For this review, take the finished solid that the model builds, in its own axes (mm). Face numbers are marked on the shaded views. A direction names the side the tool comes from. Give positions to 0.01 mm unless a question says otherwise; leave off trailing zeros. Write each loop counter-clockwise with the first axis right and the second up, starting at its lowest first coordinate (ties: lowest second). Pieces come first, ordered by that corner, then holes. Notation, with made-up numbers: (68.5, -27) -> (80.5, -27) arc R22 ccw to (80.5, -19) -> close; hole circle Ø4 at (21.25, -31.75). An arc over 180 degrees is marked (long way). Return JSON: item names as keys, results as strings.
from build123d import *

# Parameters (mm, degrees)
EKSTR_ZYON_NCE1_DEPTH = 50
IZIM2_R               = 3
KES_EKSTR_ZYON1_DEPTH = 78
IZIM3_R               = 0.5
KES_EKSTR_ZYON2_DEPTH = 22
IZIM4_R               = 6
KES_EKSTR_ZYON3_DEPTH = 22


with BuildPart() as part:
    # Çizim1 → Ekstrüzyon-İnce1 (new body)
    with BuildSketch(Plane.XY):
        with BuildLine():
            Line((0, 0), (0, 29))
            ThreePointArc((0, 29), (0.292893219, 29.707106781), (1, 30))
            Line((1, 30), (57, 30))
            ThreePointArc((57, 30), (57.707106781, 29.707106781), (58, 29))
            Line((58, 29), (58, 0))
            Line((58, 0), (57, 0))
            Line((57, 0), (57, 29))
            Line((57, 29), (1, 29))
            Line((1, 29), (1, 0))
            Line((1, 0), (0, 0))
        make_face()
    extrude(amount=EKSTR_ZYON_NCE1_DEPTH)

    # Çizim2 → Kes-Ekstrüzyon1 (cut)
    with BuildSketch(Plane(origin=(58, 0, 0), x_dir=(0, 0, -1), z_dir=(1, 0, 0))):
        with Locations((-36.75, 14.5)):
            Circle(IZIM2_R)
        with Locations((-13.25, 14.5)):
            Circle(IZIM2_R)
    extrude(amount=-KES_EKSTR_ZYON1_DEPTH, mode=Mode.SUBTRACT)

    # Çizim3 → Kes-Ekstrüzyon2 (cut)
    with BuildSketch(Plane.ZY):
        with Locations((46.926319902, 2.636193895)):
            Circle(IZIM3_R)
    extrude(amount=-KES_EKSTR_ZYON2_DEPTH, mode=Mode.SUBTRACT)

    # Çizim4 → Kes-Ekstrüzyon3 (cut)
    with BuildSketch(Plane.ZY):
        with Locations((36.75, 14.5)):
            Circle(IZIM4_R)
    extrude(amount=-KES_EKSTR_ZYON3_DEPTH, mode=Mode.SUBTRACT)


solid = part.part
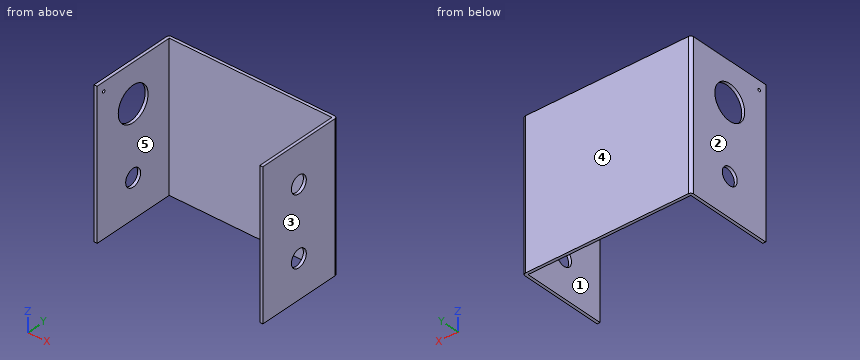
1. The part is to be moulded in two halves that separate along X. For the marked faces 1, 2 and 3, say which applies: +X half, -X half, draft (parallel to the pull), parting line (faces both ways), or undercut.
Results found:
{"face 1": "undercut", "face 2": "-X half", "face 3": "+X half"}
2. For pin 1 (1.5 mm diameter, centred on x = 22, z = 10.5, fed in from -Y), flat-tipped, find the tip position at first contact; note if it passes through.
Results found:
{"pin 1": "stops at y = 29"}
3. Add section C-C, the plane z = 13.25. State the section outline as (x, y) points, plus the area to 3 significant figures.
Results found:
{"outline": "(0, 0) -> (1, 0) -> (1, 11.5) -> (0, 11.5) -> close; (0, 17.5) -> (1, 17.5) -> (1, 29) -> (57, 29) -> (57, 17.5) -> (58, 17.5) -> (58, 29) arc R1 ccw to (57, 30) -> (1, 30) arc R1 ccw to (0, 29) -> close; (57, 0) -> (58, 0) -> (58, 11.5) -> (57, 11.5) -> close", "area": "104 mm²"}
4. For the marked faces 4 and 5, list the 3-axis set-ups (+Z, -Z, +X, -X, +Y, -Y) from which the entire face can be reached by the end or side of a thin tool; tool diameter is ignored.
Results found:
{"face 4": "+Z, -Z, +X, -X, +Y", "face 5": "+Z, -Z, -Y"}
5. Add section D-D, the plane z = 30. State the section outline as (x, y) points.
Results found:
{"outline": "(0, 0) -> (1, 0) -> (1, 29) -> (57, 29) -> (57, 0) -> (58, 0) -> (58, 29) arc R1 ccw to (57, 30) -> (1, 30) arc R1 ccw to (0, 29) -> close"}
6. Add section B-B, the plane z = 36.75. State the section outline as (x, y) points, plus the area to 3 significant figures.
Results found:
{"outline": "(0, 0) -> (1, 0) -> (1, 8.5) -> (0, 8.5) -> close; (0, 20.5) -> (1, 20.5) -> (1, 29) -> (57, 29) -> (57, 17.5) -> (58, 17.5) -> (58, 29) arc R1 ccw to (57, 30) -> (1, 30) arc R1 ccw to (0, 29) -> close; (57, 0) -> (58, 0) -> (58, 11.5) -> (57, 11.5) -> close", "area": "97.6 mm²"}
7. Add section A-A, the plane y = 14.5. State the section outline as (x, z) points.
Results found:
{"outline": "(0, 0) -> (1, 0) -> (1, 10.25) -> (0, 10.25) -> close; (0, 16.25) -> (1, 16.25) -> (1, 30.75) -> (0, 30.75) -> close; (0, 42.75) -> (1, 42.75) -> (1, 50) -> (0, 50) -> close; (57, 0) -> (58, 0) -> (58, 10.25) -> (57, 10.25) -> close; (57, 16.25) -> (58, 16.25) -> (58, 33.75) -> (57, 33.75) -> close; (57, 39.75) -> (58, 39.75) -> (58, 50) -> (57, 50) -> close"}
8. To check wall thickness, follow probe 1 along X at (y, z) = (2, 3.5); probe 2 along Y at (x, z) = (38, 36.5); probe 3 along Y at (x, z) = (57.85, 13.25). State the ranges of each line that lie inside material, in increasing order.
Results found:
{"probe 1": "x = 0 to 1, 57 to 58", "probe 2": "y = 29 to 30", "probe 3": "y = 0 to 11.5, 17.5 to 29.53"}
